from build123d import *

# Parameters (mm, degrees)
F0_W     = 31.75
F0_H     = 38.1
F1_DEPTH = 50.8
F3_DEPTH = 50.801
F4_W     = 25.4
F4_H     = 19.05
F5_DEPTH = 31.751


with BuildPart() as f1:
    # F0 (on Right) → F1 (new body)
    with BuildSketch(Plane.YZ):
        with Locations((-7.991497, 19.05)):
            Rectangle(F0_W, F0_H)
    extrude(amount=F1_DEPTH)

    # F2 (on face) → F3 (cut, through all)
    with BuildSketch(Plane(origin=(0, 0, 0), x_dir=(0, -1, 0), z_dir=(-1, 0, 0))):
        with BuildLine():
            Line((23.866497, 38.1), (-1.533503, 38.1))
            ThreePointArc((-1.533503, 38.1), (4.905563, 19.139066), (23.866497, 12.7))
            Line((23.866497, 12.7), (23.866497, 38.1))
        make_face()
    extrude(amount=-F3_DEPTH, mode=Mode.SUBTRACT)

    # F4 (on face) → F5 (cut, through all)
    with BuildSketch(Plane(origin=(0, 7.883503, 0), x_dir=(-1, 0, 0), z_dir=(0, 1, 0))):
        with Locations((-25.4, 28.575)):
            Rectangle(F4_W, F4_H)
    extrude(amount=-F5_DEPTH, mode=Mode.SUBTRACT)


solid = f1.part
The model under review builds one solid part; all positions refer to its coordinate system, in mm. A direction names the side the tool comes from. Coordinates: 2 decimals unless noted, no trailing zeros. Write each loop counter-clockwise with the first axis right and the second up, starting at its lowest first coordinate (ties: lowest second). Pieces come first, ordered by that corner, then holes. Notation, with made-up numbers: (37, 23) -> (52, 23) arc R26 ccw to (52, 56) -> close; hole circle Ø5 at (-25, 79.5). An arc over 180 degrees is marked (long way). Answer in a Markdown table with one row per item.
1. Draft analysis for pull direction X (two halves, no side actions). For faces 3 (the flat face through (25, -8, 0)), 4 (the flat face through (26, 2, 19.05)), 5 (the flat face through (50.8, -5, 15)), state which applies: +X half, -X half, draft (parallel to the pull), parting line (faces both ways), or undercut.
Answers below:
| item | result |
|---|---|
| face 3 | draft |
| face 4 | undercut |
| face 5 | +X half |
2. We need section B-B, the plane x = 41. State the section outline as (y, z) points.
Answers below:
| item | result |
|---|---|
| outline | (-23.87, 0) -> (7.88, 0) -> (7.88, 38.1) -> (1.53, 38.1) arc R22.64 cw to (-23.87, 12.7) -> close |
3. We need section C-C, the plane y = -0.5. State the section outline as (x, z) points.
Answers below:
| item | result |
|---|---|
| outline | (0, 0) -> (50.8, 0) -> (50.8, 25.36) -> (38.1, 25.36) -> (38.1, 19.05) -> (12.7, 19.05) -> (12.7, 25.36) -> (0, 25.36) -> close |
4. For faces 1 (the flat face through (12.7, 4, 26)), 2 (the flat face through (25, 7.884, 15)), list the 3-axis set-ups (+Z, -Z, +X, -X, +Y, -Y) from which the entire face can be reached by the end or side of a thin tool; tool diameter is ignored.
Answers below:
| item | result |
|---|---|
| face 1 | +Z, +Y, -Y |
| face 2 | +Z, -Z, +X, -X, +Y |
5. We need section A-A, the plane z = 30. State the section outline as (x, y) points.
Answers below:
| item | result |
|---|---|
| outline | (0, 1.13) -> (12.7, 1.13) -> (12.7, 7.88) -> (0, 7.88) -> close; (38.1, 1.13) -> (50.8, 1.13) -> (50.8, 7.88) -> (38.1, 7.88) -> close |
6. Wall thickness on probe 1 along X at (y, z) = (4.5, 28); probe 2 along Z at (x, y) = (33.5, 4); probe 3 along Z at (x, y) = (43.5, -18): over which ranges is each line inside the solid? List them lowest first. Write a range as [from, to].
Answers below:
| item | result |
|---|---|
| probe 1 | x = [0, 12.7], [38.1, 50.8] |
| probe 2 | z = [0, 19.05] |
| probe 3 | z = [0, 12.7] |
7. Clearance check with flat-ended pins moving along their axes: pin 1 Ø8 at (x, z) = (38.5, 34) entering from -Y; pin 2 Ø10.5 at (x, y) = (27.5, 2) entering from +Z; pin 3 Ø4 at (x, y) = (28.5, -19) entering from +Z. State where each tip first meets the part, or that it passes through.
Answers below:
| item | result |
|---|---|
| pin 1 | stops at y = 1.13 |
| pin 2 | stops at z = 19.05 |
| pin 3 | stops at z = 12.85 |
8. We need section D-D, the plane x = 34. State the section outline as (y, z) points, and give its area (3 significant figures).
Answers below:
| item | result |
|---|---|
| outline | (-23.87, 0) -> (7.88, 0) -> (7.88, 19.05) -> (-5, 19.05) arc R22.64 cw to (-23.87, 12.7) -> close |
| area | 514 mm^2 |
